The model under review builds one solid part; all positions refer to its coordinate system, in mm. Round coordinates to 2 decimals unless told otherwise and drop trailing zeros. Order: outer loops, then holes, each group sorted by start corner. A loop starts at its lowest first (then second) coordinate and runs counter-clockwise, first axis right, second up. Notation, with made-up numbers: M 43,1 L 99,1 A21 cw 99,11 Z; hole C -26.5,25 d6. An arc over 180 degrees is marked long. One line per item, written item: value. Start each with the question number.
from build123d import *

# Parameters (mm, degrees)
SKETCH2_R            = 11
CUT_EXTRUDE1_DEPTH   = 33.124756808
M3_CLEARANCE_HOLE1_D = 3.4


with BuildPart() as part:
    # Sketch1 → Revolve1 (revolve)
    with BuildSketch(Plane.XY, mode=Mode.PRIVATE) as revolve1_sk:
        Polygon((9, 0), (11, 0), (11, 8), (13, 8), (13, 0), (22, 0), (22, -2), (9, -2), align=None)
    revolve(revolve1_sk.sketch.rotate(Axis((0, 17.954019247, 0), (0, -1, 0)), 90), axis=Axis((0, 17.954019247, 0), (0, -1, 0)))

    # Sketch2 → Cut-Extrude1 (cut, through all)
    with BuildSketch(Plane(origin=(0, 0, 0), x_dir=(1, 0, 0), z_dir=(0, 1, 0))):
        with Locations(Location((0, 0, 0), (0, 0, 270))):
            Circle(SKETCH2_R)
    extrude(amount=-CUT_EXTRUDE1_DEPTH, mode=Mode.SUBTRACT)

    # M3 Clearance Hole1 (through all)
    with Locations(Plane(origin=(0, 0, 0), x_dir=(1, 0, 0), z_dir=(0, 1, 0))):
        with Locations((0, 17.5), (17.5, 0), (0, -17.5), (-17.5, 0)):
            Hole(M3_CLEARANCE_HOLE1_D / 2)


solid = part.part
Item 1: Clearance check with flat-ended pins moving along their axes: P1, Ø5, axis at x = -8, y = 2, coming from the -Z side; P2, Ø6, axis at x = 12, y = 0.5, coming from the -Z side; P3, Ø1.5, axis at y = 4.5, z = 0.5, coming from the +X side. State where each tip first meets the part, or that it passes through.
Item 2: Wall thickness on L1, parallel to X at y = 5.25, z = 0; L2, parallel to Y at x = -18, z = 11; L3, parallel to Z at x = -3, y = 2: over which ranges is each line inside the solid? List them lowest first.
Item 3: Consider section C-C, the plane z = -17.5. Give the boundary of the cut face in (x, y), then the cut area to 3 significant figures.
Item 4: Consider section A-A, the plane z = 0. Give the boundary of the cut face in (x, y), then the cut area to 3 significant figures.
Item 5: Consider section D-D, the plane x = 6. Give the boundary of the cut face in (y, z), then the cut area to 3 significant figures.
Item 6: Consider section B-B, the plane x = 0. Give the boundary of the cut face in (y, z), then the cut area to 3 significant figures.
Item 7: The part is to be moulded in two halves that separate along Z. For faces 1 (the cylindrical face through (0.221, -1.014, 15.814)), 2 (the cylindrical face through (7.91, 3.944, -10.316)), 3 (the flat face through (9.5, 0, -9.5)), say which applies: pulls with the +Z half, pulls with the -Z half, needs draft (parallel to the pull), parting line crosses it, or undercut.
Computed:
1. P1: stops at z = -21.02
1. P2: stops at z = -20.06
1. P3: stops at x = 13
2. L1: x = -13 to -11, 11 to 13
2. L2: y = -2 to 0
2. L3: z = -12.65 to -10.58, 10.58 to 12.65
3. outline: M -13.33,-2 L -1.7,-2 L -1.7,0 L -13.33,0 Z; M 1.7,-2 L 13.33,-2 L 13.33,0 L 1.7,0 Z
3. area: 46.5 mm^2
4. outline: M -22,-2 L -19.2,-2 L -19.2,0 L -22,0 Z; M -15.8,-2 L -11,-2 L -11,8 L -13,8 L -13,0 L -15.8,0 Z; M 11,-2 L 15.8,-2 L 15.8,0 L 13,0 L 13,8 L 11,8 Z; M 19.2,-2 L 22,-2 L 22,0 L 19.2,0 Z
4. area: 62.4 mm^2
5. outline: M -2,-21.17 L 0,-21.17 L 0,-11.53 L 8,-11.53 L 8,-9.22 L -2,-9.22 Z; M -2,9.22 L 8,9.22 L 8,11.53 L 0,11.53 L 0,21.17 L -2,21.17 Z
5. area: 84.8 mm^2
6. outline: M -2,-22 L 0,-22 L 0,-19.2 L -2,-19.2 Z; M -2,-15.8 L 0,-15.8 L 0,-13 L 8,-13 L 8,-11 L -2,-11 Z; M -2,11 L 8,11 L 8,13 L 0,13 L 0,15.8 L -2,15.8 Z; M -2,19.2 L 0,19.2 L 0,22 L -2,22 Z
6. area: 62.4 mm^2
7. face 1: undercut
7. face 2: parting line crosses it
7. face 3: needs draft
